Verification items for the finished model (mm, model axes). A direction names the side the tool comes from. Coordinates: 2 decimals unless noted, no trailing zeros. Write each loop counter-clockwise with the first axis right and the second up, starting at its lowest first coordinate (ties: lowest second). Pieces come first, ordered by that corner, then holes. Notation, with made-up numbers: (-13, 69) -> (-7, 69) arc R29 cw to (-7, 100) -> close; hole circle Ø2 at (74, -36). An arc over 180 degrees is marked (long way). Answer in a Markdown table with one row per item.
```python
from build123d import *

# Parameters (mm, degrees)
SKETCH_2_W      = 49.600012207
SKETCH_2_H      = 22.800017408
SKETCH_2_W_2    = 10.900003052
SKETCH_2_H_2    = 18.800017408
SKETCH_2_W_3    = 6
SKETCH_2_W_4    = 10.900003051
EXTRUDE_1_DEPTH = 1
SKETCH_4_W      = 49.600012207
SKETCH_4_H      = 1
EXTRUDE_2_DEPTH = 2
SKETCH_5_W      = 49.600012207
SKETCH_5_H      = 1
EXTRUDE_3_DEPTH = 15
SKETCH_6_W      = 1
SKETCH_6_H      = 17.650008704
EXTRUDE_6_DEPTH = 1
SKETCH_7_W      = 2
SKETCH_7_H      = 2
EXTRUDE_7_DEPTH = 2
SKETCH_8_W      = 2
SKETCH_8_H      = 1
EXTRUDE_8_DEPTH = 2
CHAMFER_1_SIZE  = 2


with BuildPart() as part:
    # Эскиз2 → Бобышка-Вытянуть1 (new body)
    with BuildSketch(Plane.XY):
        with Locations((22.600006104, 10.200008704)):
            Rectangle(SKETCH_2_W, SKETCH_2_H)
        with Locations((10.150004578, 10.200008704)):
            Rectangle(SKETCH_2_W_2, SKETCH_2_H_2, mode=Mode.SUBTRACT)
        with Locations((22.600006104, 10.200008704)):
            Rectangle(SKETCH_2_W_3, SKETCH_2_H_2, mode=Mode.SUBTRACT)
        with Locations((35.05000763, 10.200008704)):
            Rectangle(SKETCH_2_W_4, SKETCH_2_H_2, mode=Mode.SUBTRACT)
    extrude(amount=EXTRUDE_1_DEPTH)

    # Эскиз4 → Бобышка-Вытянуть2 (add)
    with BuildSketch(Plane.XZ.offset(1.2)):
        with Locations((22.600006104, 0.5)):
            Rectangle(SKETCH_4_W, SKETCH_4_H)
    extrude(amount=EXTRUDE_2_DEPTH)

    # Эскиз5 → Бобышка-Вытянуть3 (add)
    with BuildSketch(Plane(origin=(0, 0, 0), x_dir=(-1, 0, 0), z_dir=(0, 0, -1))):
        with Locations((-22.600006104, -2.7)):
            Rectangle(SKETCH_5_W, SKETCH_5_H)
    extrude(amount=EXTRUDE_3_DEPTH)

    # Эскиз6 → Бобышка-Вытянуть6 (add)
    with BuildSketch(Plane.ZY.offset(2.2)):
        with Locations((0.5, 12.775013056)):
            Rectangle(SKETCH_6_W, SKETCH_6_H)
        Polygon((1, 3.950008704), (0, 3.950008704), (0, -2.2), (-15, -2.2), (-15, -3.2), (1, -3.2), align=None)
        Polygon((0, -2.2), (0, 3.950008704), (-1, 3.950008704), (-15, 6.184703554), (-15, -2.2), align=None)
    extrude_6 = extrude(amount=EXTRUDE_6_DEPTH)

    # Зеркальное отражение1: Бобышка-Вытянуть6 across plane
    add(extrude_6.mirror(Plane.ZY.offset(-22.600006104)))

    # Эскиз7 → Бобышка-Вытянуть7 (add)
    with BuildSketch(Plane(origin=(0, 0, 0), x_dir=(-1, 0, 0), z_dir=(0, 0, -1))):
        with Locations((-44.400012207, 18.600017408)):
            Rectangle(SKETCH_7_W, SKETCH_7_H)
        with Locations((-0.8, 18.600017408)):
            Rectangle(SKETCH_7_W, SKETCH_7_H)
    extrude(amount=EXTRUDE_7_DEPTH)

    # Эскиз8 → Бобышка-Вытянуть8 (add)
    with BuildSketch(Plane(origin=(0, 19.600017408, 0), x_dir=(1, 0, 0), z_dir=(0, 1, 0))):
        with Locations((0.8, 1.5)):
            Rectangle(SKETCH_8_W, SKETCH_8_H)
        with Locations((44.400012207, 1.5)):
            Rectangle(SKETCH_8_W, SKETCH_8_H)
    extrude(amount=EXTRUDE_8_DEPTH)

    # Фаска1
    chamfer_1_edges = [part.edges().sort_by_distance(p)[0] for p in [
        (0.8, 17.600017408, -2),
        (44.400012207, 17.600017408, -2),
    ]]
    chamfer(chamfer_1_edges, length=CHAMFER_1_SIZE - 0.0001)  # a hair under: the kernel refuses the full size


solid = part.part
```
1. Section check C-C, the plane y = -1.5. Record the boundary of the cut face in (x, z), plus the area to 3 significant figures.
Geometry says:
| item | result |
|---|---|
| outline | (-3.2, -15) -> (-2.2, -15) -> (-2.2, 0) -> (47.4, 0) -> (47.4, -15) -> (48.4, -15) -> (48.4, 1) -> (-3.2, 1) -> close |
| area | 81.6 mm^2 |
2. Depth check by flat-ended pin: P1, Ø2, axis at x = 16, y = 14.5, coming from the -Z side; P2, Ø4, axis at y = 18, z = -3.5, coming from the +X side; P3, Ø0.6, axis at x = 44, y = 20.5, coming from the -Z side. Enter the tip coordinate at first touch or a pass-through.
Geometry says:
| item | result |
|---|---|
| P1 | z = 0 |
| P2 | through |
| P3 | z = -2 |
3. Thickness scan on line 1 (X direction, y = 2.5, z = -4); line 2 (Y direction, x = 8, z = -11.75); line 3 (Z direction, x = 27.5, y = 18). Record the ranges inside material, lowest first. Write a range as from..to.
Geometry says:
| item | result |
|---|---|
| line 1 | -3.2..-2.2, 47.4..48.4 |
| line 2 | -3.2..-2.2 |
| line 3 | 0..1 |
4. Section check A-A, the plane y = 6.75. Record the boundary of the cut face in (x, z), plus the area to 3 significant figures.
Geometry says:
| item | result |
|---|---|
| outline | (-3.2, 0) -> (4.7, 0) -> (4.7, 1) -> (-3.2, 1) -> close; (15.6, 0) -> (19.6, 0) -> (19.6, 1) -> (15.6, 1) -> close; (25.6, 0) -> (29.6, 0) -> (29.6, 1) -> (25.6, 1) -> close; (40.5, 0) -> (48.4, 0) -> (48.4, 1) -> (40.5, 1) -> close |
| area | 23.8 mm^2 |
5. Section check B-B, the plane x = 11.5. Record the boundary of the cut face in (y, z).
Geometry says:
| item | result |
|---|---|
| outline | (-3.2, -15) -> (-2.2, -15) -> (-2.2, 0) -> (0.8, 0) -> (0.8, 1) -> (-3.2, 1) -> close; (19.6, 0) -> (21.6, 0) -> (21.6, 1) -> (19.6, 1) -> close |
6. Tool access check on faces 1 (the flat face through (47.4, 1, -8)), 2 (the flat face through (35, 0.8, 0.5)), 3 (the flat face through (1, 21, -1)), 4 (the flat face through (44.4, 18.6, -1)). Record the directions out of +Z, -Z, +X, -X, +Y, -Y that give a thin tool (end or side, any length) a straight path to the whole face; none if there is none.
Geometry says:
| item | result |
|---|---|
| face 1 | -Z, +Y |
| face 2 | +Z, -Z |
| face 3 | +X, -X, +Y |
| face 4 | -Z, +X, -X |
7. Mould release check, pull along X, two halves, no side actions. Record for faces 5 (the flat face through (15.6, 10.1, 0.5)), 6 (the flat face through (44, 21, -2)), 7 (the flat face through (10.1, 0.8, 0.5)), 8 (the flat face through (-3.2, 3, -7)): released by +X, released by -X, zero draft, split by the parting line, or undercut.
Geometry says:
| item | result |
|---|---|
| face 5 | undercut |
| face 6 | zero draft |
| face 7 | undercut |
| face 8 | released by -X |
